Here's how the part is built. I have some questions about the finished solid (model axes, mm). A direction names the side the tool comes from. Coordinates: 2 decimals unless noted, no trailing zeros. Order: outer loops, then holes, each group sorted by start corner. A loop starts at its lowest first (then second) coordinate and runs counter-clockwise, first axis right, second up. Notation, with made-up numbers: (28, -11.5) - (55, -11.5) arc R25 ccw to (55, 14.5) - close; hole circle Ø6 at (33.25, -21). An arc over 180 degrees is marked (long way). Answer as CSV lines item,"result". Start each with the question number.
Item 1: Imagine slicing it at A-A on x = 11. List the corners of the cut face in (y, z) for me.
Item 2: We'd pull the mould along Y, two halves only. Please class faces 5 (the face through (-10.375, 26, 40)), 6 (the face through (-1.503, 21.681, 35.226)), 7 (the face through (2.16, 23.74, 20.87)), 8 (the face through (25, 38.1, 3)): pulls with the +Y half, pulls with the -Y half, needs draft (parallel to the pull), parting line crosses it, or undercut.
Item 3: On a 3-axis mill with a long thin cutter (end or side, diameter ignored), from which of +Z, -Z, +X, -X, +Y, -Y can I reach the whole of each face in a straight line? I mean faces 1 (the face through (2.3, 7.3, 51.5)), 2 (the face through (-10.78, 33.82, 40.93)), 3 (the face through (-2.975, 37, 39)), 4 (the face through (25, 31.75, 3)). Say none if no direction works.
Item 4: Imagine slicing it at C-C on y = 24.5. Count the separate pieces of the cut face and the enclosed holes in it, and give its area (3 significant figures).
Item 5: Imagine slicing it at B-B on z = 63.5. List the corners of the cut face in (x, y) for me (1 decimal).
Item 6: I need wall thicknesses on line 1 (Y direction, x = -3.4, z = 39.5) (3 decimals); line 2 (X direction, y = 16, z = 42.5) (1 decimal); line 3 (Y direction, x = -5, z = 39). Which ranges of each line are inside material? Lowest first, please.
Item 7: I'm going to push flat-ended pins straight in: pin 1 (2 mm diameter, centred on x = 41.5, y = 5, fed in from +Z); pin 2 (10 mm diameter, centred on y = 36.572, z = 39.5, fed in from -X) (3 decimals); pin 3 (3 mm diameter, centred on y = 36.5, z = 38.5, fed in from -X) (3 decimals); pin 4 (5 mm diameter, centred on y = 36.5, z = 39.5, fed in from +X). Where does each tip first touch, or does it pass through?
from build123d import *

# Parameters (mm, degrees)
BOSS_EXTRUDE1_DEPTH   = 50.8
SKETCH2_W             = 41.275
SKETCH2_H             = 25.4
CUT_EXTRUDE1_DEPTH    = 95.399536545
SKETCH3_W             = 41.275
SKETCH3_H             = 63.5
CUT_EXTRUDE2_DEPTH    = 95.399536545
SKETCH4_R             = 2.75
CUT_EXTRUDE3_DEPTH    = 95.399536545
FILLET1_R             = 2.54
FILLET3_DEPTH         = 4.7625
FILLET3_START         = 46.0375
FILLET3_2_DEPTH       = 4.7625
F_8_CLEARANCE_HOLE1_D = 4.4958
BOSS_EXTRUDE2_START   = -4.7625
SKETCH9_W             = 7.2
SKETCH9_H             = 41.275
BOSS_EXTRUDE2_DEPTH   = 15.9375
SKETCH10_R            = 3.1
CUT_EXTRUDE4_DEPTH    = 0.8
SKETCH10_3_R          = 2.4
CUT_EXTRUDE5_DEPTH    = 7.2
CUT_EXTRUDE9_START    = -7.2
SKETCH10_4_R          = 3.1
SKETCH10_4_R_2        = 2.4
CUT_EXTRUDE9_DEPTH    = 1
FILLET4_R             = 3.6


with BuildPart() as part:
    # Sketch1 → Boss-Extrude1 (new body)
    with BuildSketch(Plane(origin=(0, 0, 0), x_dir=(0, 0, -1), z_dir=(1, 0, 0))):
        Polygon((0, 0), (0, 38.1), (-6.35, 38.1), (-69.85, 6.35), (-69.85, 0), align=None)
        Polygon((-55.650968343, 6.35), (-6.35, 6.35), (-6.35, 31.000484171), align=None, mode=Mode.SUBTRACT)
    extrude(amount=BOSS_EXTRUDE1_DEPTH)

    # Sketch2 → Cut-Extrude1 (cut, through all)
    with BuildSketch(Plane.XY.offset(69.85)):
        with Locations((25.4, 19.05)):
            Rectangle(SKETCH2_W, SKETCH2_H)
    extrude(amount=-CUT_EXTRUDE1_DEPTH, mode=Mode.SUBTRACT)

    # Sketch3 → Cut-Extrude2 (cut, through all)
    with BuildSketch(Plane.XZ):
        with Locations((25.4, 38.1)):
            Rectangle(SKETCH3_W, SKETCH3_H)
    extrude(amount=-CUT_EXTRUDE2_DEPTH, mode=Mode.SUBTRACT)

    # Sketch4 → Cut-Extrude3 (cut, through all)
    with BuildSketch(Plane(origin=(50.8, 0, 0), x_dir=(0, 0, -1), z_dir=(1, 0, 0))):
        with Locations((-63.5, 4.572)):
            Circle(SKETCH4_R)
    extrude(amount=-CUT_EXTRUDE3_DEPTH, mode=Mode.SUBTRACT)

    # Fillet1
    fillet1_edges = [part.edges().sort_by_distance(p)[0] for p in [
        (2.38125, 6.35, 69.85),
        (2.38125, 0, 69.85),
        (48.41875, 0, 69.85),
        (48.41875, 6.35, 69.85),
    ]]
    fillet(fillet1_edges, radius=FILLET1_R)

    # Fillet3: read off the stored shape, not the designer's step
    # Fillet3 outline → Fillet3 (add)
    with BuildSketch(Plane.YZ):
        with BuildLine():
            ThreePointArc((7.62, 6.35), (6.721974388, 6.721974388), (6.35, 7.62))
            Line((6.35, 7.62), (6.35, 6.35))
            Line((6.35, 6.35), (7.62, 6.35))
        make_face()
        with BuildLine():
            Line((6.35, 55.650968343), (6.35, 50.271162011))
            ThreePointArc((6.35, 50.271162011), (7.328213791, 51.507188228), (8.755922533, 50.839123278))
            Line((8.755922533, 50.839123278), (6.35, 55.650968343))
        make_face()
        with BuildLine():
            ThreePointArc((30.081503538, 8.187961266), (30.025907532, 6.952321488), (28.945581006, 6.35))
            Line((28.945581006, 6.35), (31.000484171, 6.35))
            Line((31.000484171, 6.35), (30.081503538, 8.187961266))
        make_face()
    extrude(amount=FILLET3_DEPTH)

    # Fillet3 2 outline → Fillet3 2 (add)
    with BuildSketch(Plane.YZ.offset(FILLET3_START)):
        with BuildLine():
            ThreePointArc((7.62, 6.35), (6.721974388, 6.721974388), (6.35, 7.62))
            Line((6.35, 7.62), (6.35, 6.35))
            Line((6.35, 6.35), (7.62, 6.35))
        make_face()
        with BuildLine():
            Line((6.35, 55.650968343), (6.35, 50.271162011))
            ThreePointArc((6.35, 50.271162011), (7.328213791, 51.507188228), (8.755922533, 50.839123278))
            Line((8.755922533, 50.839123278), (6.35, 55.650968343))
        make_face()
        with BuildLine():
            ThreePointArc((30.081503538, 8.187961266), (30.025907532, 6.952321488), (28.945581006, 6.35))
            Line((28.945581006, 6.35), (31.000484171, 6.35))
            Line((31.000484171, 6.35), (30.081503538, 8.187961266))
        make_face()
    extrude(amount=FILLET3_2_DEPTH)

    # #8 Clearance Hole1 (through all)
    with Locations(Plane.XY.offset(6.35)):
        with Locations((14.9225, 34.925), (35.8775, 34.925), (14.9225, 3.175), (35.8775, 3.175)):
            Hole(F_8_CLEARANCE_HOLE1_D / 2)

    # Sketch9 → Boss-Extrude2 (add)
    with BuildSketch(Plane.ZY.offset(BOSS_EXTRUDE2_START)):
        with Locations((39.5, 20.6375)):
            Rectangle(SKETCH9_W, SKETCH9_H)
    extrude(amount=BOSS_EXTRUDE2_DEPTH)

    # Sketch10 → Cut-Extrude4 (cut)
    with BuildSketch(Plane.ZY.offset(11.175)):
        with Locations((39.5, 36.572)):
            Circle(SKETCH10_R)
        with Locations((39.5, 28.572)):
            Circle(SKETCH10_R)
        with Locations((39.5, 20.572)):
            Circle(SKETCH10_R)
    extrude(amount=-CUT_EXTRUDE4_DEPTH, mode=Mode.SUBTRACT)

    # Sketch10<3> → Cut-Extrude5 (cut)
    with BuildSketch(Plane.ZY.offset(11.175)):
        with Locations((39.5, 20.572)):
            Circle(SKETCH10_3_R)
        with Locations((39.5, 36.572)):
            Circle(SKETCH10_3_R)
        with Locations((39.5, 28.572)):
            Circle(SKETCH10_3_R)
    extrude(amount=-CUT_EXTRUDE5_DEPTH, mode=Mode.SUBTRACT)

    # Sketch10<4> → Cut-Extrude9 (cut)
    # profile 1 of 5: a face of its own
    with BuildSketch(Plane.ZY.offset(11.175).offset(CUT_EXTRUDE9_START)):
        with Locations((39.5, 28.572)):
            Circle(SKETCH10_4_R)
        with Locations((39.5, 28.572)):
            Circle(SKETCH10_4_R_2, mode=Mode.SUBTRACT)
    # profile 2 of 5: a face of its own
    with BuildSketch(Plane.ZY.offset(11.175).offset(CUT_EXTRUDE9_START)):
        with Locations((39.5, 28.572)):
            Circle(SKETCH10_4_R_2)
    # profile 3 of 5: a face of its own
    with BuildSketch(Plane.ZY.offset(11.175).offset(CUT_EXTRUDE9_START)):
        with Locations((39.5, 20.572)):
            Circle(SKETCH10_4_R)
        with Locations((39.5, 20.572)):
            Circle(SKETCH10_4_R_2, mode=Mode.SUBTRACT)
    # profile 4 of 5: a face of its own
    with BuildSketch(Plane.ZY.offset(11.175).offset(CUT_EXTRUDE9_START)):
        with Locations((39.5, 20.572)):
            Circle(SKETCH10_4_R_2)
    # profile 5 of 5: a face of its own
    with BuildSketch(Plane.ZY.offset(11.175).offset(CUT_EXTRUDE9_START)):
        with Locations((39.5, 36.572)):
            Circle(SKETCH10_4_R)
    extrude(amount=-CUT_EXTRUDE9_DEPTH, mode=Mode.SUBTRACT)

    # Fillet4
    fillet4_edges = [part.edges().sort_by_distance(p)[0] for p in [
        (-3.20625, 41.275, 43.1),
        (-3.20625, 41.275, 35.9),
        (2.38125, 12.625484171, 43.1),
        (0, 16.175242086, 43.1),
        (2.38125, 19.725, 43.1),
        (2.38125, 16.225484171, 35.9),
        (0, 19.775242086, 35.9),
        (2.38125, 23.325, 35.9),
    ]]
    fillet(fillet4_edges, radius=FILLET4_R - 0.0001)  # a hair under: the kernel refuses the full size


solid = part.part
Responses:
1,outline,"(0, 0) - (6.35, 0) - (6.35, 6.35) - (0, 6.35) - close; (31.75, 0) - (38.1, 0) - (38.1, 6.35) - (31.75, 6.35) - close"
2,face 5,"undercut"
2,face 6,"needs draft"
2,face 7,"undercut"
2,face 8,"pulls with the +Y half"
3,face 1,"+X, -X"
3,face 2,"-X"
3,face 3,"none"
3,face 4,"+Z, -Z"
4,separate pieces,"4"
4,enclosed holes,"0"
4,area,"324 mm^2"
5,outline,"(0, 0) - (4.8, 0) - (4.8, 1.8) - (0, 1.8) - close; (0, 7.3) - (4.8, 7.3) - (4.8, 9.5) - (0, 9.5) - close; (46, 0) - (50.8, 0) - (50.8, 1.8) - (46, 1.8) - close; (46, 7.3) - (50.8, 7.3) - (50.8, 9.5) - (46, 9.5) - close"
6,line 1,"y = 0 to 17.472, 23.672 to 25.472, 31.672 to 33.472, 39.672 to 41.275"
6,line 2,"x = -11.2 to 4.8, 46 to 50.8"
6,line 3,"y = 0 to 18.22, 22.92 to 26.22, 30.92 to 34.22, 38.92 to 41.24"
7,pin 1,"stops at z = 6.35"
7,pin 2,"stops at x = -11.175"
7,pin 3,"stops at x = -10.375"
7,pin 4,"stops at x = 4.76"
